```python
from build123d import *

# Parameters (mm, degrees)
BOX_W             = 0.5
BOX_H             = 6
BOX_DEPTH         = 12
CYLINDER005_R     = 3
CYLINDER005_DEPTH = 12
CYLINDER002_R     = 15
CYLINDER002_DEPTH = 2
CYLINDER003_R     = 6
CYLINDER003_DEPTH = 2.5
CYLINDER004_R     = 0.25
CYLINDER004_DEPTH = 2
CYLINDER_R        = 15
CYLINDER_DEPTH    = 2
CYLINDER001_R     = 10
CYLINDER001_DEPTH = 5.5


with BuildPart() as obj1:
    # Box → Box (new body)
    with BuildSketch(Plane(origin=(2.5, -3, 0), x_dir=(1, 0, 0), z_dir=(0, 0, 1))):
        with Locations((0.25, 3)):
            Rectangle(BOX_W, BOX_H)
    extrude(amount=BOX_DEPTH)


with BuildPart() as shafthole:
    # Cylinder005 → Cylinder005 (new body)
    with BuildSketch(Plane.XY):
        Circle(CYLINDER005_R)
    extrude(amount=CYLINDER005_DEPTH)

    # Cut: cut obj1
    add(obj1.part, mode=Mode.SUBTRACT)


with BuildPart() as bottom:
    # Cylinder002 → Cylinder002 (new body)
    with BuildSketch(Plane.XY.offset(2.5)):
        Circle(CYLINDER002_R)
    extrude(amount=CYLINDER002_DEPTH)


with BuildPart() as standoff:
    # Cylinder003 → Cylinder003 (new body)
    with BuildSketch(Plane.XY):
        Circle(CYLINDER003_R)
    extrude(amount=CYLINDER003_DEPTH)


with BuildPart() as obj2:
    # Cylinder004 → Cylinder004 (new body)
    with BuildSketch(Plane(origin=(11, 0, 10), x_dir=(1, 0, 0), z_dir=(0, 0, 1))):
        Circle(CYLINDER004_R)
    extrude(amount=CYLINDER004_DEPTH)


with BuildPart() as obj3:
    # Cylinder → Cylinder (new body)
    with BuildSketch(Plane.XY.offset(10)):
        Circle(CYLINDER_R)
    extrude(amount=CYLINDER_DEPTH)

    # Cut001: cut obj2
    add(obj2.part, mode=Mode.SUBTRACT)


with BuildPart() as body:
    # Cylinder001 → Cylinder001 (new body)
    with BuildSketch(Plane.XY.offset(4.5)):
        Circle(CYLINDER001_R)
    extrude(amount=CYLINDER001_DEPTH)

    # Fusion: union Bottom, Standoff, obj3
    add(bottom.part)
    add(standoff.part)
    add(obj3.part)

    # Cut002: cut ShaftHole
    add(shafthole.part, mode=Mode.SUBTRACT)


solid = body.part
```
Source: CAD feature listing. Evaluate the final solid. Frame: model axes, mm. A direction names the side the tool comes from. Coordinates: 2 decimals unless noted, no trailing zeros. Loops run counter-clockwise (first coordinate to the right, second up) from the corner with the lowest first, then second, coordinate; pieces in that order, holes last. Notation, with made-up numbers: M -32,61 L 9,61 A10 cw 9,72 Z; hole C -22,50 d5. An arc over 180 degrees is marked long. Use a Markdown table: item, result. Add a question column.
Q1. Access query for faces 4 (the cylindrical face through (-2.17, -9.76, 7.21)), 5 (the flat face through (2.5, 0, 6)), 6 (the cylindrical face through (-6, 0, 1)). Directions: +Z, -Z, +X, -X, +Y, -Y. A direction counts if a zero-diameter tool reaches every point of the face in a straight line with its end or side. Return the directions, or none.
Q2. Section query B-B, the plane y = 13. Return loops of the section in (x, z), and give its area (3 significant figures).
Q3. Draft query along Z for faces 1 (the cylindrical face through (-3, 0, 6)), 2 (the flat face through (3, 0, 12)), 3 (the flat face through (3, -10, 4.5)). Return one class per face: pulls with the +Z half, pulls with the -Z half, needs draft (parallel to the pull), parting line crosses it, or undercut.
Q4. Material intervals for L1, parallel to Z at x = 11, y = -7; L2, parallel to Y at x = 0, z = 7; L3, parallel to Z at x = 2.5, y = -9.5, sorted ascending.
Q5. Section query C-C, the plane z = 5.5. Return loops of the section in (x, y), and give its area (3 significant figures).
Q6. Section query D-D, the plane x = -8.75. Return loops of the section in (y, z).
Q7. Section query A-A, the plane x = 0. Return loops of the section in (y, z).
Q8. First-contact query: pin 1 (1.5 mm diameter, centred on x = -1.5, z = 6, fed in from -Y); pin 2 (1 mm diameter, centred on x = 2, z = 3.5, fed in from -Y); pin 3 (5 mm diameter, centred on y = 6.5, z = 3, fed in from +X). Flat tips, straight axial feed; report the tip coordinate or a pass-through.
Result:
| question | item | result |
|---|---|---|
| 1 | face 4 | none |
| 1 | face 5 | +Z, -Z |
| 1 | face 6 | -Z |
| 2 | outline | M -7.48,2.5 L 7.48,2.5 L 7.48,4.5 L -7.48,4.5 Z; M -7.48,10 L 7.48,10 L 7.48,12 L -7.48,12 Z |
| 2 | area | 59.9 mm2 |
| 3 | face 1 | needs draft |
| 3 | face 2 | pulls with the +Z half |
| 3 | face 3 | undercut |
| 4 | L1 | z = 2.5 to 4.5, 10 to 12 |
| 4 | L2 | y = -10 to -3, 3 to 10 |
| 4 | L3 | z = 2.5 to 12 |
| 5 | outline | C 0,0 d20; hole M 2.5,-1.66 L 2.5,1.66 A3 ccw long Z |
| 5 | area | 287 mm2 |
| 6 | outline | M -12.18,2.5 L 12.18,2.5 L 12.18,4.5 L 4.84,4.5 L 4.84,10 L 12.18,10 L 12.18,12 L -12.18,12 L -12.18,10 L -4.84,10 L -4.84,4.5 L -12.18,4.5 Z |
| 7 | outline | M -15,2.5 L -6,2.5 L -6,0 L -3,0 L -3,12 L -15,12 L -15,10 L -10,10 L -10,4.5 L -15,4.5 Z; M 3,0 L 6,0 L 6,2.5 L 15,2.5 L 15,4.5 L 10,4.5 L 10,10 L 15,10 L 15,12 L 3,12 Z |
| 8 | pin 1 | stops at y = -9.97 |
| 8 | pin 2 | stops at y = -14.92 |
| 8 | pin 3 | stops at x = 14.46 |
